```python
from build123d import *

# Parameters (mm, degrees)
SKETCH1_W             = 50
SKETCH1_H             = 150
BOSS_EXTRUDE1_DEPTH   = 12
M5_TAPPED_HOLE1_D     = 4.2
M5_TAPPED_HOLE1_DEPTH = 10
M5_TAPPED_HOLE1_TIP   = 1.2618073
M5_TAPPED_HOLE2_D     = 4.2
M5_TAPPED_HOLE2_DEPTH = 10
M5_TAPPED_HOLE2_TIP   = 1.2618073
CHAMFER1_SIZE         = 30
CHAMFER2_SIZE         = 2


with BuildPart() as part:
    # Sketch1 → Boss-Extrude1 (new body)
    with BuildSketch(Plane.XY):
        with Locations((-27.5, 38.28125)):
            Rectangle(SKETCH1_W, SKETCH1_H)
    extrude(amount=BOSS_EXTRUDE1_DEPTH)

    # M5 Tapped Hole1
    with Locations(Plane.ZY.offset(52.5)):
        with Locations((6, 98.28125), (6, 43.28125), (6, -11.71875)):
            Hole(M5_TAPPED_HOLE1_D / 2, depth=M5_TAPPED_HOLE1_DEPTH)
            with Locations((0, 0, -(M5_TAPPED_HOLE1_DEPTH + M5_TAPPED_HOLE1_TIP / 2))):  # 118° drill point
                Cone(0, M5_TAPPED_HOLE1_D / 2, M5_TAPPED_HOLE1_TIP, mode=Mode.SUBTRACT)

    # M5 Tapped Hole2
    with Locations(Plane(origin=(0, -36.71875, 0), x_dir=(-1, 0, 0), z_dir=(0, -1, 0))):
        with Locations((46.5, -6), (8.5, -6)):
            Hole(M5_TAPPED_HOLE2_D / 2, depth=M5_TAPPED_HOLE2_DEPTH)
            with Locations((0, 0, -(M5_TAPPED_HOLE2_DEPTH + M5_TAPPED_HOLE2_TIP / 2))):  # 118° drill point
                Cone(0, M5_TAPPED_HOLE2_D / 2, M5_TAPPED_HOLE2_TIP, mode=Mode.SUBTRACT)

    # Chamfer1
    chamfer1_edges = [part.edges().sort_by_distance(p)[0] for p in [
        (-2.5, 113.28125, 6),
    ]]
    chamfer(chamfer1_edges, length=CHAMFER1_SIZE)

    # Chamfer2
    chamfer2_edges = [part.edges().sort_by_distance(p)[0] for p in [
        (-52.5, -36.71875, 6),
    ]]
    chamfer(chamfer2_edges, length=CHAMFER2_SIZE)


solid = part.part
```
Build history of the part. All positions in model axes, mm. A direction names the side the tool comes from. Round coordinates to 2 decimals unless told otherwise and drop trailing zeros. Write each loop counter-clockwise with the first axis right and the second up, starting at its lowest first coordinate (ties: lowest second). Pieces come first, ordered by that corner, then holes. Notation, with made-up numbers: (10, 39) - (34, 39) arc R7 cw to (34, 49) - close; hole circle Ø3 at (49.5, -17). An arc over 180 degrees is marked (long way). Write each question's results on one line, items separated by ' | '. Start each with the question number.
Item 1: Mould opens along Y. For faces 4 (the face through (-41.457, 97.925, 5.921)), 5 (the face through (-43, 113.281, 6)), 6 (the face through (-28, 39, 12)) say: pulls with the +Y half, pulls with the -Y half, needs draft (parallel to the pull), parting line crosses it, or undercut.
Item 2: Saw through at A-A (z = 10.25). Write the cut outline in (x, y), and give its area (3 significant figures).
Item 3: Saw through at B-B (x = -24). Write the cut outline in (y, z).
Item 4: Wall check: L1, parallel to Y at x = -49.75, z = 6; L2, parallel to Y at x = -47.25, z = 6; L3, parallel to Z at x = -8, y = -33. Give the ranges that are in metal, low to high. Write a range as [from, to].
Item 5: Drop flat-ended pins along their axis: P1, Ø4, axis at x = -46.5, z = 6, coming from the -Y side; P2, Ø4, axis at y = 98.28, z = 6, coming from the -X side; P3, Ø6.5, axis at x = -8.5, z = 6, coming from the +Y side. Give the stop position or say it passes through.
Item 6: Which spindle directions (+Z, -Z, +X, -X, +Y, -Y) get a long thin tool onto all of the face, cutting with end or side? Do faces 1 (the face through (-47.43, 41.231, 6.455)), 2 (the face through (-44.56, -31.65, 6.8)), 3 (the face through (-52.5, 38, 6)). Say none if no direction does.
Results are:
1) face 4: undercut | face 5: pulls with the +Y half | face 6: needs draft
2) outline: (-52.5, -34.72) - (-50.5, -36.72) - (-2.5, -36.72) - (-2.5, 83.28) - (-32.5, 113.28) - (-52.5, 113.28) - close | area: 7,050 mm²
3) outline: (-36.72, 0) - (104.78, 0) - (104.78, 12) - (-36.72, 12) - close
4) L1: y = [-36.72, -13.82], [-9.62, 41.18], [45.38, 96.18], [100.38, 113.28] | L2: y = [-25.91, -13.82], [-9.62, 41.18], [45.38, 96.18], [100.38, 113.28] | L3: z = [0, 3.96], [8.04, 12]
5) P1: stops at y = -26.66 | P2: stops at x = -42.44 | P3: stops at y = 92.53
6) face 1: -X | face 2: -Y | face 3: +Z, -Z, -X, +Y, -Y
